Answer from the drawing. Dimensions are ordinates in mm from the lowest x, y and z of the part. Coordinates: 2 decimals unless noted, no trailing zeros. Order: outer loops, then holes, each group sorted by start corner. A loop starts at its lowest first (then second) coordinate and runs counter-clockwise, first axis right, second up. Notation, with made-up numbers: (-3.75, 25) - (38.25, 25) arc R29 cw to (38.25, 48) - close; hole circle Ø7 at (32.5, -37.75). An arc over 180 degrees is marked (long way). Answer as a JSON object with one key per item and string values. Group by question number.
1) Section A-A (z = 1) is taken. Give the vertices of the cut face in (x, y).
2) Section C-C (y = 2.5) is taken. Give the vertices of the cut face in (x, z).
3) This flat-tipped pin is pushed along its axis until it touches: P1, Ø1, axis at x = 1.5, y = 8, coming from the -Z side. Where does it stop, or does it pass through?
4) Section B-B (y = 5.25) is taken. Give the vertices of the cut face in (x, z).
5) Find the intervals of material crossed by line 1 along Y through (x, z) = (0.65, 1.05); line 2 along X through (y, z) = (5, 1.05), in increasing order.
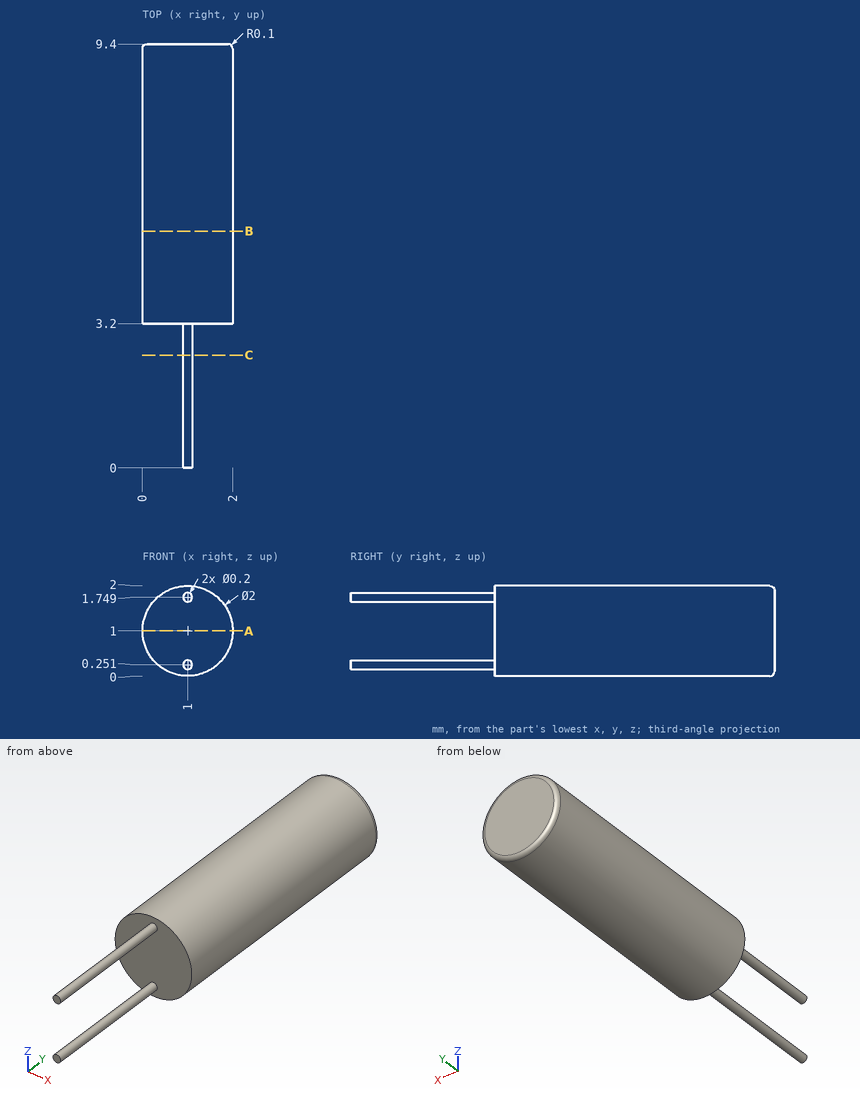
Report:
{
 "1": {"outline": "(0, 3.2) - (2, 3.2) - (2, 9.3) arc R0.1 ccw to (1.9, 9.4) - (0.1, 9.4) arc R0.1 ccw to (0, 9.3) - close"},
 "2": {"outline": "circle Ø0.2 at (1, 0.25); circle Ø0.2 at (1, 1.75)"},
 "3": {"P1": "stops at z = 0"},
 "4": {"outline": "circle Ø2 at (1, 1)"},
 "5": {"line 1": "y = 3.2 to 9.4", "line 2": "x = 0 to 2"}
}
